```python
from build123d import *

# Parameters (mm, degrees)
SKETCH1_R           = 5
BOSS_EXTRUDE1_DEPTH = 5
SKETCH1_3_R         = 5
BOSS_EXTRUDE2_DEPTH = 10


with BuildPart() as part:
    # Sketch1 → Boss-Extrude1 (new body)
    with BuildSketch(Plane.XY):
        with BuildLine():
            ThreePointArc((-7.07496458, -7.067168895), (6.531960096, -7.571888622), (8.028425575, 5.961911001))
            add(Edge.make_bspline(
                [(6.054624404, 592.041261198), (-154.861931166, 445.129888812), (-96.296929143, 163.306236232), (8.028425575, 5.961911001)],
                knots=[0, 0, 0, 0, 1, 1, 1, 1], degree=3))
            ThreePointArc((6.054624404, 592.041261198), (7.812843537, 606.241752628), (-6.425366596, 607.662549452))
            add(Edge.make_bspline(
                [(-6.425366596, 607.662549452), (-277.843168438, 277.304372569), (-7.07496458, -7.067168895)],
                knots=[0, 0, 0, 1, 1, 1], degree=2))
        make_face()
        Circle(SKETCH1_R, mode=Mode.SUBTRACT)
        with Locations((-100, 200)):
            Circle(SKETCH1_R, mode=Mode.SUBTRACT)
        with Locations((0, 600)):
            Circle(SKETCH1_R, mode=Mode.SUBTRACT)
    boss_extrude1 = extrude(amount=BOSS_EXTRUDE1_DEPTH)

    # Sketch1<3> → Boss-Extrude2 (add)
    with BuildSketch(Plane.XY):
        Circle(SKETCH1_3_R)
    boss_extrude2 = extrude(amount=BOSS_EXTRUDE2_DEPTH)

    # Mirror1: Boss-Extrude1, Boss-Extrude2 across Front Plane
    add(boss_extrude1.mirror(Plane.XY))
    add(boss_extrude2.mirror(Plane.XY))


solid = part.part
```
Can you work these out from the model? Positions are in its coordinate system, mm. A direction names the side the tool comes from. Coordinates: 2 decimals unless noted, no trailing zeros.
1) I need wall thicknesses on probe 1 along Y at (x, z) = (0, 1.85); probe 2 along Z at (x, y) = (-94, 289); probe 3 along X at (y, z) = (600, -3.15). Which ranges of each line are inside material? Lowest first, please.
2) Which directions (+Z, -Z, +X, -X, +Y, -Y) give clear straight access to the entire face, cutting with the end or side of a thin tool? Please do faces 1 (the flat face through (0, 0, -10)), 2 (the cylindrical face through (-1.08, -4.88, 7.46)), 3 (the cylindrical face through (-1.08, -4.88, -7.46)).
3) For pin 1 (9 mm diameter, centred on x = 0, y = 600, fed in from +Z); pin 2 (5 mm diameter, centred on x = -76.5, y = 508.5, fed in from +Z); pin 3 (10 mm diameter, centred on x = -99, z = -6.5, fed in from -Y); pin 4 (12 mm diameter, centred on x = -109.5, z = -3, fed in from -Y), each with a flat end and sliding along its axis, tell me the tip position at first contact or that it passes through.
Completed:
1. probe 1: y = -10 to 18.46, 586.35 to 595, 605 to 610
1. probe 2: z = -5 to 5
1. probe 3: x = -12.65 to -5, 5 to 10
2. face 1: -Z, +X, -X, +Y, -Y
2. face 2: +Z
2. face 3: -Z
3. pin 1: passes through
3. pin 2: stops at z = 5
3. pin 3: stops at y = 109.49
3. pin 4: stops at y = 127.3
